from build123d import *

# Parameters (mm, degrees)
SKETCH1_R           = 14.2875
BOSS_EXTRUDE1_DEPTH = 0.79375
CUT_EXTRUDE1_DEPTH  = 2.5875


with BuildPart() as part:
    # Sketch1 → Boss-Extrude1 (new body, symmetric)
    with BuildSketch(Plane.XY):
        Circle(SKETCH1_R)
    extrude(amount=BOSS_EXTRUDE1_DEPTH, both=True)

    # Sketch2 → Cut-Extrude1 (cut, through all)
    with BuildSketch(Plane(origin=(0, 0, -0.79375), x_dir=(-1, 0, 0), z_dir=(0, 0, -1))):
        with BuildLine():
            ThreePointArc((-7.329682086, 8.352449747), (-5.130117272, 8.885623765), (-3.568592622, 10.523915761))
            ThreePointArc((-3.568592622, 10.523915761), (0, 12.7), (3.568592622, 10.523915761))
            ThreePointArc((3.568592622, 10.523915761), (5.130117272, 8.885623765), (7.329682086, 8.352449747))
            ThreePointArc((7.329682086, 8.352449747), (10.998522628, 6.35), (10.898274707, 2.171466014))
            ThreePointArc((10.898274707, 2.171466014), (10.260234545, 0), (10.898274707, -2.171466014))
            ThreePointArc((10.898274707, -2.171466014), (10.998522628, -6.35), (7.329682086, -8.352449747))
            ThreePointArc((7.329682086, -8.352449747), (5.130117272, -8.885623765), (3.568592622, -10.523915761))
            ThreePointArc((3.568592622, -10.523915761), (0, -12.7), (-3.568592622, -10.523915761))
            ThreePointArc((-3.568592622, -10.523915761), (-5.130117272, -8.885623765), (-7.329682086, -8.352449747))
            ThreePointArc((-7.329682086, -8.352449747), (-10.998522628, -6.35), (-10.898274707, -2.171466014))
            ThreePointArc((-10.898274707, -2.171466014), (-10.260234545, 0), (-10.898274707, 2.171466014))
            ThreePointArc((-10.898274707, 2.171466014), (-10.998522628, 6.35), (-7.329682086, 8.352449747))
        make_face()
    extrude(amount=-CUT_EXTRUDE1_DEPTH, mode=Mode.SUBTRACT)


solid = part.part
Verification items for the finished model (mm, model axes). Coordinates: 2 decimals unless noted, no trailing zeros. Order: outer loops, then holes, each group sorted by start corner. A loop starts at its lowest first (then second) coordinate and runs counter-clockwise, first axis right, second up. Notation, with made-up numbers: (1, 51.25) -> (44, 51.25) arc R17 cw to (44, 71.25) -> close; hole circle Ø1 at (30.25, 22.25). An arc over 180 degrees is marked (long way). Use CSV: the item, a comma, the result in double quotes. Start each with the question number.
Q1. Thickness scan on line 1 along Y through (x, z) = (-0.25, -0.1); line 2 along Y through (x, z) = (0.75, -0.3); line 3 along X through (y, z) = (5.25, -0.2). Record the ranges inside material, lowest first.
Q2. Section check A-A, the plane y = 0. Record the cut outline in (x, z).
Q3. Section check B-B, the plane x = 0. Record the cut outline in (y, z), and give its area (3 significant figures).
Q4. Section check C-C, the plane z = -0.2. Record the cut outline in (x, y) (1 decimal).
Q5. Depth check by flat-ended pin: P1, Ø5, axis at x = -7.5, y = -5, coming from the -Z side. Enter the tip coordinate at first touch or a pass-through.
Returned:
1,line 1,"y = -14.29 to -12.69, 12.69 to 14.29"
1,line 2,"y = -14.27 to -12.63, 12.63 to 14.27"
1,line 3,"x = -13.29 to -11.43, 11.43 to 13.29"
2,outline,"(-14.29, -0.79) -> (-10.26, -0.79) -> (-10.26, 0.79) -> (-14.29, 0.79) -> close; (10.26, -0.79) -> (14.29, -0.79) -> (14.29, 0.79) -> (10.26, 0.79) -> close"
3,outline,"(-14.29, -0.79) -> (-12.7, -0.79) -> (-12.7, 0.79) -> (-14.29, 0.79) -> close; (12.7, -0.79) -> (14.29, -0.79) -> (14.29, 0.79) -> (12.7, 0.79) -> close"
3,area,"5.04 mm^2"
4,outline,"circle Ø28.6 at (0, 0); hole (-10.9, -2.2) arc R4 ccw to (-7.3, -8.4) arc R4 cw to (-3.6, -10.5) arc R4 ccw to (3.6, -10.5) arc R4 cw to (7.3, -8.4) arc R4 ccw to (10.9, -2.2) arc R4 cw to (10.9, 2.2) arc R4 ccw to (7.3, 8.4) arc R4 cw to (3.6, 10.5) arc R4 ccw to (-3.6, 10.5) arc R4 cw to (-7.3, 8.4) arc R4 ccw to (-10.9, 2.2) arc R4 cw to start"
5,P1,"passes through"
